from build123d import *

# Parameters (mm, degrees)
PAD035_DEPTH    = 77
SKETCH115_R     = 3.1
POCKET071_DEPTH = 30
SKETCH116_R     = 4.3
POCKET072_DEPTH = 100
CHAMFER014_SIZE = 12
PAD036_DEPTH    = 2
SKETCH118_W     = 30
SKETCH118_H     = 16
POCKET073_DEPTH = 8
CHAMFER023_SIZE = 0.5


with BuildPart() as part:
    # Sketch114 → Pad035 (new body)
    with BuildSketch(Plane.YZ):
        Polygon((-47, 203.208383528), (-19, 203.208383528), (-22.5, 189.708383528), (22.5, 189.708383528), (19, 203.208383528), (47, 203.208383528), (47, 174.470931), (-47, 174.470931), align=None)
    extrude(amount=PAD035_DEPTH)

    # Sketch115 (on Face3 of Pad035) → Pocket071 (cut)
    with BuildSketch(Plane(origin=(0, 0, 189.708383528), x_dir=(0, -1, 0), z_dir=(0, 0, 1))):
        with Locations((0, 47)):
            Circle(SKETCH115_R)
    extrude(amount=-POCKET071_DEPTH, mode=Mode.SUBTRACT)

    # Sketch116 (on Face2 of Pocket071) → Pocket072 (cut)
    with BuildSketch(Plane(origin=(0, -47, 0), x_dir=(0, 0, -1), z_dir=(0, -1, 0))):
        with Locations((-182.470931, 65)):
            Circle(SKETCH116_R)
    extrude(amount=-POCKET072_DEPTH, mode=Mode.SUBTRACT)

    # Chamfer014
    chamfer014_edges = [part.edges().sort_by_distance(p)[0] for p in [
        (38.5, 47, 203.208384),
        (38.5, -47, 203.208384),
    ]]
    chamfer(chamfer014_edges, length=CHAMFER014_SIZE)

    # Sketch117 (on Face2 of Chamfer014) → Pad036 (join)
    with BuildSketch(Plane(origin=(0, 0, 0), x_dir=(0, 1, 0), z_dir=(-1, 0, 0))):
        Polygon((-47, -174.470931), (47, -174.470931), (47, -191.208383528), (35, -203.208383528), (-35, -203.208383528), (-47, -191.208383528), align=None)
    extrude(amount=PAD036_DEPTH)

    # Sketch118 (on Face15 of Pad036) → Pocket073 (cut)
    with BuildSketch(Plane.ZX.offset(47)):
        with Locations((189.470931, 65)):
            Rectangle(SKETCH118_W, SKETCH118_H)
        with Locations((189.470931, 12)):
            Rectangle(SKETCH118_W, SKETCH118_H)
    extrude(amount=-POCKET073_DEPTH, mode=Mode.SUBTRACT)

    # Chamfer023
    chamfer023_edges = [part.edges().sort_by_distance(p)[0] for p in [
        (73, 43, 195.208384),
        (57, 43, 195.208384),
        (57, 47, 182.839657),
        (73, 47, 182.839657),
        (20, 43, 195.208384),
        (4, 43, 195.208384),
        (4, 47, 182.839657),
        (20, 47, 182.839657),
        (47, 3.1, 174.470931),
        (65, 39, 186.770931),
        (65, -47, 186.770931),
    ]]
    chamfer(chamfer023_edges, length=CHAMFER023_SIZE)


with BuildPart() as part_1:
    # Body027 placement: moved
    add(part.part.moved(Location((-37, 0, 113))))


solid = part_1.part
Could you check a few things on this model? Use its own coordinates, in mm. A direction names the side the tool comes from. Give positions to 0.01 mm unless a question says otherwise; leave off trailing zeros. Order: outer loops, then holes, each group sorted by start corner. A loop starts at its lowest first (then second) coordinate and runs counter-clockwise, first axis right, second up.
Item 1: I'm going to push flat-ended pins straight in: pin 1 (22.5 mm diameter, centred on x = 5.5, y = 5.5, fed in from +Z); pin 2 (5 mm diameter, centred on x = 26, z = 296, fed in from +Y); pin 3 (4 mm diameter, centred on x = 9.5, z = 308.5, fed in from +Y). Where does each tip first touch, or does it pass through?
Item 2: If we section it at C-C, the plane y = -30.5: Write out the boundary of the cut face in (x, z).
Item 3: If we section it at D-D, the plane x = -27: Write out the boundary of the cut face in (y, z).
Item 4: If we section it at B-B, the plane x = 28: Write out the boundary of the cut face in (y, z).
Item 5: If we mould it in two halves opening along Z, with no side actions, what happens to faces 1 (the face through (38, 47, 296)), 2 (the face through (19.747, 42.882, 307.978)), 3 (the face through (0.961, 20.774, 309.364))? For each: pulls with the +Z half, pulls with the -Z half, needs draft (parallel to the pull), parting line crosses it, or undercut.
Item 6: For faces 4 (the face through (-33, 43, 297)), 5 (the face through (-39, 1, 302)), 6 (the face through (1.05, 39.75, 311.46)), 7 (the face through (-16.746, 42.882, 307.978)), which set-ups out of +Z, -Z, +X, -X, +Y, -Y let a thin tool reach every point of the face, with its end or its side?
Item 7: If we section it at A-A, the plane y = 0: Write out the boundary of the cut face in (x, z).
Item 8: I need wall thicknesses on line 1 (X direction, y = 0, z = 297.5); line 2 (X direction, y = -2, z = 292.75); line 3 (Y direction, x = 25.5, z = 299.75). Which ranges of each line are inside material? Lowest first, please.
Values:
1. pin 1: stops at z = 302.71
1. pin 2: stops at y = 38.77
1. pin 3: stops at y = 44.71
2. outline: (-39, 287.47) - (40, 287.47) - (40, 316.21) - (-39, 316.21) - close; hole circle Ø8.6 at (28, 295.47)
3. outline: (-47, 287.47) - (39, 287.47) - (39, 312.21) - (35, 316.21) - (19, 316.21) - (22.5, 302.71) - (-22.5, 302.71) - (-19, 316.21) - (-35, 316.21) - (-47, 304.21) - close
4. outline: (-47, 287.47) - (39, 287.47) - (39, 290.67) - (38.5, 291.17) - (-46.5, 291.17) - (-47, 290.67) - close; (-47, 300.27) - (-46.5, 299.77) - (38.5, 299.77) - (39, 300.27) - (39, 312.21) - (35, 316.21) - (19, 316.21) - (22.5, 302.71) - (-22.5, 302.71) - (-19, 316.21) - (-35, 316.21) - (-47, 304.21) - close
5. face 1: needs draft
5. face 2: pulls with the +Z half
5. face 3: undercut
6. face 4: +Z, -Z, +Y
6. face 5: +Z, -Z, -X, +Y, -Y
6. face 6: +Z, +X, -X, +Y
6. face 7: +Z, +Y
7. outline: (-39, 287.47) - (6.4, 287.47) - (6.9, 287.97) - (6.9, 302.71) - (-37, 302.71) - (-37, 316.21) - (-39, 316.21) - close; (13.1, 287.97) - (13.6, 287.47) - (40, 287.47) - (40, 302.71) - (13.1, 302.71) - close; hole circle Ø8.6 at (28, 295.47)
8. line 1: x = -39 to 6.9, 13.1 to 24.21, 31.79 to 40
8. line 2: x = -39 to 7.63, 12.37 to 24.67, 31.33 to 40
8. line 3: y = -47 to 39
